Part model, mm, in its own coordinate system. A direction names the side the tool comes from. Round coordinates to 2 decimals unless told otherwise and drop trailing zeros. Loops run counter-clockwise (first coordinate to the right, second up) from the corner with the lowest first, then second, coordinate; pieces in that order, holes last. Notation, with made-up numbers: M 81,16.25 L 85,16.25 A19 cw 85,24.25 Z; hole C 65,36 d9. An arc over 180 degrees is marked long. Put each result on its own line as item: value. Start each with the question number.
```python
from build123d import *

# Parameters (mm, degrees)
BOSS_EXTRUDE2_DEPTH  = 3
SKETCH3_R            = 4.5
CUT_EXTRUDE3_DEPTH   = 8
SKETCH4_R            = 5
CUT_EXTRUDE4_DEPTH   = 1.5
BOSS_EXTRUDE3_DEPTH  = 20.5
BOSS_EXTRUDE4_DEPTH  = 38
BOSS_EXTRUDE5_DEPTH  = 17.5
SKETCH10_R           = 1.5
BOSS_EXTRUDE6_DEPTH  = 3
BOSS_EXTRUDE6_TAPER  = 15
SKETCH11_R           = 2
CUT_EXTRUDE6_DEPTH   = 3
CUT_EXTRUDE6_TAPER   = 6
SKETCH12_W           = 12.8
SKETCH12_H           = 5
BOSS_EXTRUDE11_DEPTH = 3
SKETCH13_W           = 34
SKETCH13_H           = 5
BOSS_EXTRUDE12_DEPTH = 3
SKETCH9_R            = 1
CUT_EXTRUDE5_DEPTH   = 5
SKETCH15_W           = 4
SKETCH15_H           = 2.5
CUT_EXTRUDE7_DEPTH   = 10
SKETCH16_W           = 4
SKETCH16_H           = 5
BOSS_EXTRUDE13_DEPTH = 14.5
SKETCH17_R           = 1.5
BOSS_EXTRUDE14_DEPTH = 3
BOSS_EXTRUDE14_TAPER = 17


with BuildPart() as part:
    # Sketch1 → Boss-Extrude2 (new body, symmetric)
    with BuildSketch(Plane.XY):
        with BuildLine():
            Line((-44.599094606, 4.924384255), (-20.111639684, 23.933975293))
            ThreePointArc((-20.111639684, 23.933975293), (-18.64459039, 24.726101678), (-17, 25))
            Line((-17, 25), (17, 25))
            ThreePointArc((17, 25), (18.64459039, 24.726101678), (20.111639684, 23.933975293))
            Line((20.111639684, 23.933975293), (44.599094606, 4.924384255))
            ThreePointArc((44.599094606, 4.924384255), (47.095170256, -3.430752773), (40, -8.5))
            Line((40, -8.5), (-40, -8.5))
            ThreePointArc((-40, -8.5), (-47.095170256, -3.430752773), (-44.599094606, 4.924384255))
        make_face()
    extrude(amount=BOSS_EXTRUDE2_DEPTH, both=True)

    # Sketch3 → Cut-Extrude3 (cut)
    with BuildSketch(Plane(origin=(0, 0, -3), x_dir=(-1, 0, 0), z_dir=(0, 0, -1))):
        with Locations((-39.987497786, -1.00001042)):
            Circle(SKETCH3_R)
    cut_extrude3 = extrude(amount=-CUT_EXTRUDE3_DEPTH, mode=Mode.SUBTRACT)

    # Sketch4 → Cut-Extrude4 (cut)
    with BuildSketch(Plane(origin=(0, 0, -3), x_dir=(-1, 0, 0), z_dir=(0, 0, -1))):
        with Locations((-39.987497786, -1.00001042)):
            Circle(SKETCH4_R)
    cut_extrude4 = extrude(amount=-CUT_EXTRUDE4_DEPTH, mode=Mode.SUBTRACT)

    # Mirror1: Cut-Extrude3, Cut-Extrude4 across plane
    add(cut_extrude3.mirror(Plane(origin=(0, 0, 0), x_dir=(0, 0, 1), z_dir=(1, 0, 0))), mode=Mode.SUBTRACT)
    add(cut_extrude4.mirror(Plane(origin=(0, 0, 0), x_dir=(0, 0, 1), z_dir=(1, 0, 0))), mode=Mode.SUBTRACT)

    # Sketch5 → Boss-Extrude3 (add)
    with BuildSketch(Plane(origin=(0, 0, -3), x_dir=(-1, 0, 0), z_dir=(0, 0, -1))):
        Polygon((-17, 25), (17, 25), (17, 20), (2, 20), (2, -3.5), (16, -3.5), (16, -8.5), (-16, -8.5), (-16, -3.5), (-2, -3.5), (-2, 20), (-17, 20), align=None)
    extrude(amount=BOSS_EXTRUDE3_DEPTH)

    # Sketch7 → Boss-Extrude4 (add)
    with BuildSketch(Plane(origin=(0, 0, -3), x_dir=(-1, 0, 0), z_dir=(0, 0, -1))):
        with BuildLine():
            Line((17, 20), (22.575001918, 15.691897491))
            Line((22.575001918, 15.691897491), (25.641064989, 19.641486995))
            Line((25.641064989, 19.641486995), (20.111639684, 23.933975293))
            ThreePointArc((20.111639684, 23.933975293), (18.64459039, 24.726101678), (17, 25))
            Line((17, 25), (17, 20))
        make_face()
    boss_extrude4 = extrude(amount=BOSS_EXTRUDE4_DEPTH)

    # Mirror2: Boss-Extrude4 across plane
    add(boss_extrude4.mirror(Plane(origin=(0, 0, 0), x_dir=(0, 0, 1), z_dir=(1, 0, 0))))

    # Sketch8 → Boss-Extrude5 (add)
    with BuildSketch(Plane(origin=(0, 0, -23.5), x_dir=(-1, 0, 0), z_dir=(0, 0, -1))):
        Polygon((0, -8.5), (3, -8.5), (2, -3.5), (-2, -3.5), (-3, -8.5), align=None)
    extrude(amount=BOSS_EXTRUDE5_DEPTH)

    # Sketch10 → Boss-Extrude6 (add)
    with BuildSketch(Plane(origin=(0, 0, -41), x_dir=(-1, 0, 0), z_dir=(0, 0, -1))):
        with Locations((21, 20.079456047)):
            Circle(SKETCH10_R)
        with Locations((0, -6)):
            Circle(SKETCH10_R)
    boss_extrude6 = extrude(amount=BOSS_EXTRUDE6_DEPTH, taper=BOSS_EXTRUDE6_TAPER)

    # Mirror3: Boss-Extrude6 across plane
    add(boss_extrude6.mirror(Plane(origin=(0, 0, 0), x_dir=(0, 0, 1), z_dir=(1, 0, 0))))

    # Sketch11 → Cut-Extrude6 (cut)
    with BuildSketch(Plane.XY.offset(3)):
        with Locations((0, 15)):
            Circle(SKETCH11_R)
        with Locations((30, 12.5)):
            Circle(SKETCH11_R)
        with Locations((-30, 12.5)):
            Circle(SKETCH11_R)
    extrude(amount=-CUT_EXTRUDE6_DEPTH, taper=CUT_EXTRUDE6_TAPER, mode=Mode.SUBTRACT)

    # Sketch12 → Boss-Extrude11 (add)
    with BuildSketch(Plane(origin=(0, 0, -23.5), x_dir=(-1, 0, 0), z_dir=(0, 0, -1))):
        with Locations((-9.6, -6)):
            Rectangle(SKETCH12_W, SKETCH12_H)
    boss_extrude11 = extrude(amount=BOSS_EXTRUDE11_DEPTH)

    # Mirror4: Boss-Extrude11 across plane
    add(boss_extrude11.mirror(Plane(origin=(0, 0, 0), x_dir=(0, 0, 1), z_dir=(1, 0, 0))))

    # Sketch13 → Boss-Extrude12 (add)
    with BuildSketch(Plane(origin=(0, 0, -23.5), x_dir=(-1, 0, 0), z_dir=(0, 0, -1))):
        with Locations((0, 22.5)):
            Rectangle(SKETCH13_W, SKETCH13_H)
    extrude(amount=BOSS_EXTRUDE12_DEPTH)

    # Sketch9 → Cut-Extrude5 (cut)
    with BuildSketch(Plane(origin=(0, 0, -23.5), x_dir=(-1, 0, 0), z_dir=(0, 0, -1))):
        with Locations((-9.85, -6)):
            Circle(SKETCH9_R)
        with Locations((-9.85, 22.2)):
            Circle(SKETCH9_R)
        with Locations((9.85, 22.2)):
            Circle(SKETCH9_R)
        with Locations((9.85, -6)):
            Circle(SKETCH9_R)
    extrude(amount=CUT_EXTRUDE5_DEPTH, mode=Mode.SUBTRACT)

    # Sketch15 → Cut-Extrude7 (cut)
    with BuildSketch(Plane.XZ.offset(8.5)):
        with Locations((-9.85, -15.82)):
            Rectangle(SKETCH15_W, SKETCH15_H)
        with Locations((9.85, -15.82)):
            Rectangle(SKETCH15_W, SKETCH15_H)
    extrude(amount=-CUT_EXTRUDE7_DEPTH, mode=Mode.SUBTRACT)

    # Sketch16 → Boss-Extrude13 (add)
    with BuildSketch(Plane(origin=(0, 0, -26.5), x_dir=(-1, 0, 0), z_dir=(0, 0, -1))):
        with Locations((0, 22.5)):
            Rectangle(SKETCH16_W, SKETCH16_H)
    extrude(amount=BOSS_EXTRUDE13_DEPTH)

    # Sketch17 → Boss-Extrude14 (add)
    with BuildSketch(Plane(origin=(0, 0, -41), x_dir=(-1, 0, 0), z_dir=(0, 0, -1))):
        with Locations((0, 22.5)):
            Circle(SKETCH17_R)
    extrude(amount=BOSS_EXTRUDE14_DEPTH, taper=BOSS_EXTRUDE14_TAPER)


solid = part.part
```
1. Drop flat-ended pins along their axis: pin 1 (2 mm diameter, centred on y = -7, z = -15.5, fed in from +X); pin 2 (1 mm diameter, centred on x = -12.5, y = 16, fed in from -Z); pin 3 (1.5 mm diameter, centred on x = -10.5, y = -7, fed in from -Z); pin 4 (6 mm diameter, centred on x = 31, z = -16, fed in from +Y). Give the stop position or say it passes through.
2. Cut at A-A, the plane z = -25. Give the cut face in (x, y) (3 decimals).
3. Cut at B-B, the plane x = -9.85. Give the cut face in (y, z), and give its area (4 significant figures).
4. Which spindle directions (+Z, -Z, +X, -X, +Y, -Y) get a long thin tool onto all of the face, cutting with end or side? Do faces 5 (the conical face through (-28.278, 13.042, 1.146)), 6 (the flat face through (0, -3.5, -32)), 7 (the flat face through (-10, -6, -14.57)), 8 (the flat face through (-19, 20, -41)), 9 (the flat face through (-19.748, 17.876, -21.734)). Say none if no direction does.
5. Cut at C-C, the plane z = -40. Give the cut face in (x, y) (3 decimals), and give its area (3 significant figures).
6. Mould opens along X. For faces 1 (the conical face through (0.22, -6.98, -42.85)), 2 (the flat face through (-7.5, -3.5, -14.6)), 3 (the flat face through (24.087, 17.639, -21.734)), 4 (the cylindrical face through (-10.39, -5.16, -24.98)) say: released by +X, released by -X, zero draft, split by the parting line, or undercut.
7. Wall check: L1, parallel to Y at x = -9.85, z = -24.2; L2, parallel to X at y = 23, z = -33; L3, parallel to X at y = 22.2, z = -24.3. Give the ranges that are in metal, low to high.
8. Cut at D-D, the plane y = 7. Give the cut face in (x, z).
Results list:
1. pin 1: stops at x = 16
1. pin 2: stops at z = -3
1. pin 3: stops at z = -26.5
1. pin 4: passes through
2. outline: M -25.641,19.641 L -22.575,15.692 L -17,20 L 17,20 L 22.575,15.692 L 25.641,19.641 L 20.112,23.934 A5.074 ccw 17,25 L -17,25 A5.074 ccw -20.112,23.934 Z; M -16,-8.5 L -3.2,-8.5 L -3.2,-3.5 L -16,-3.5 Z; M -3,-8.5 L 3,-8.5 L 2,-3.5 L -2,-3.5 Z; M 3.2,-8.5 L 16,-8.5 L 16,-3.5 L 3.2,-3.5 Z; hole C -9.85,-6 d2; hole C -9.85,22.2 d2; hole C 9.85,-6 d2; hole C 9.85,22.2 d2
3. outline: M -8.5,-26.5 L -7,-26.5 L -7,-23.5 L -5,-23.5 L -5,-26.5 L -3.5,-26.5 L -3.5,-17.07 L -8.5,-17.07 Z; M -8.5,-14.57 L -3.5,-14.57 L -3.5,-3 L 20,-3 L 20,-26.5 L 21.2,-26.5 L 21.2,-23.5 L 23.2,-23.5 L 23.2,-26.5 L 25,-26.5 L 25,3 L -8.5,3 Z
3. area: 411.5 mm^2
4. face 5: +Z
4. face 6: -Z, +X, -X
4. face 7: -Y
4. face 8: -Z
4. face 9: -Z, -Y
5. outline: M -25.641,19.641 L -22.575,15.692 L -17,20 L -17,25 A5.074 ccw -20.112,23.934 Z; M -3,-8.5 L 3,-8.5 L 2,-3.5 L -2,-3.5 Z; M -2,20 L 2,20 L 2,25 L -2,25 Z; M 17,20 L 22.575,15.692 L 25.641,19.641 L 20.112,23.934 A5.074 ccw 17,25 Z
5. area: 132 mm^2
6. face 1: split by the parting line
6. face 2: zero draft
6. face 3: released by +X
6. face 4: undercut
7. L1: y = -8.5 to -7, -5 to -3.5, 20 to 21.2, 23.2 to 25
7. L2: x = -21.31 to -17, -2 to 2, 17 to 21.31
7. L3: x = -22.35 to -10.85, -8.85 to 8.85, 10.85 to 22.35
8. outline: M -41.93,-3 L -2,-3 L -2,-23.5 L 2,-23.5 L 2,-3 L 41.93,-3 L 41.93,3 L -41.93,3 Z
